Drawing for the job (mm, zero at the part's lowest x, y, z). Round coordinates to 2 decimals unless told otherwise and drop trailing zeros. Write each loop counter-clockwise with the first axis right and the second up, starting at its lowest first coordinate (ties: lowest second). Pieces come first, ordered by that corner, then holes. Notation, with made-up numbers: (53.25, 48) -> (108.25, 48) arc R20 cw to (108.25, 84) -> close; hole circle Ø5 at (77, 39). An arc over 180 degrees is marked (long way). Answer in a Markdown table with one row per item. Add a question column.
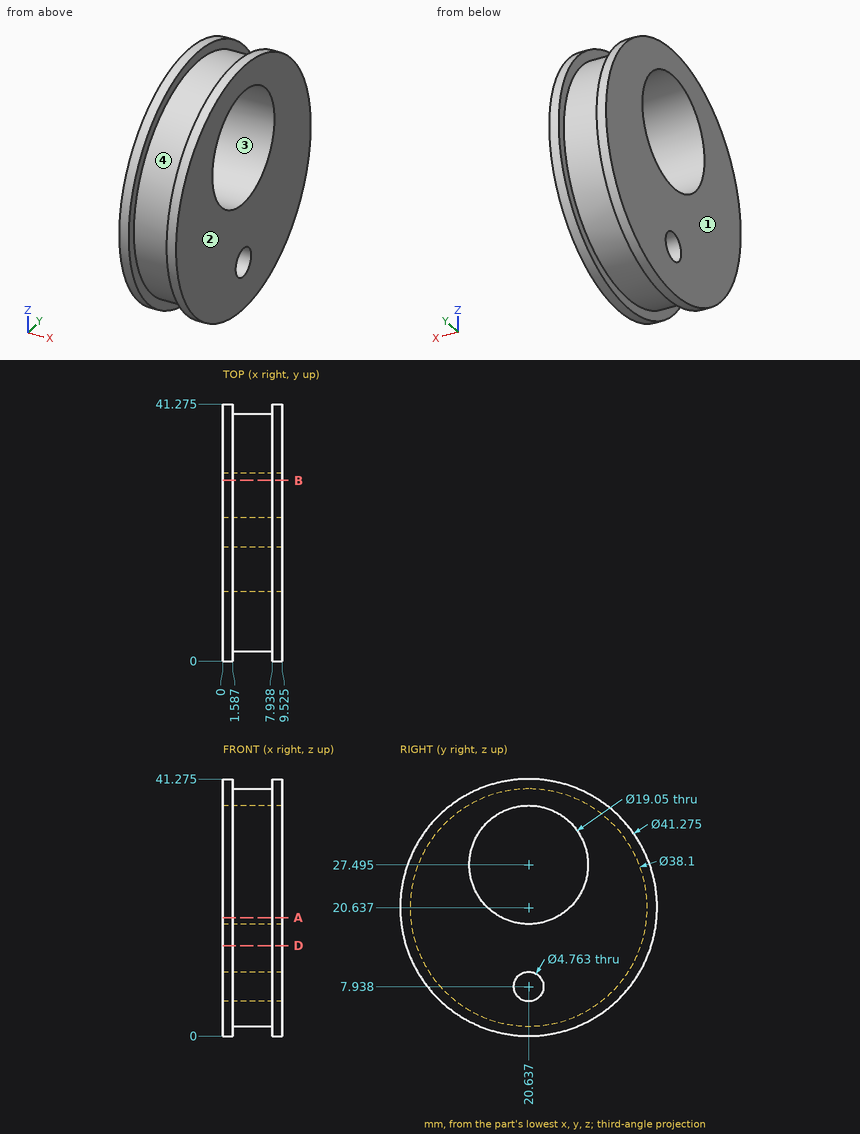
(1) Mould opens along X. For the marked faces 1, 2, 3 and 4 say: pulls with the +X half, pulls with the -X half, needs draft (parallel to the pull), parting line crosses it, or undercut.
(2) Saw through at B-B (y = 29). List the corners of the cut face in (x, z) (1 decimal), plus the area to 3 significant figures.
(3) Probe line 1 along X through (y, z) = (24, 39.5) (1 decimal); line 2 along Z through (x, y) = (2.5, 19) (1 decimal); line 3 along Y through (x, z) = (8, 9.5) (1 decimal). List the from-to ranges inside material, lowest first.
(4) Drop flat-ended pins along their axis: P1, Ø1, axis at x = 6, z = 10.5, coming from the -Y side (1 decimal); P2, Ø4, axis at x = 5.5, z = 4.5, coming from the +Y side (1 decimal); P3, Ø1, axis at x = 5, y = 8, coming from the -Z side (1 decimal). Give the stop position or say it passes through.
(5) Saw through at D-D (z = 14.5). List the corners of the cut face in (x, y) (1 decimal), plus the area to 3 significant figures.
(6) Saw through at A-A (z = 19). List the corners of the cut face in (x, y) (1 decimal).
Answer sheet:
| question | item | result |
|---|---|---|
| 1 | face 1 | pulls with the -X half |
| 1 | face 2 | pulls with the +X half |
| 1 | face 3 | needs draft |
| 1 | face 4 | undercut |
| 2 | outline | (0, 1.8) -> (1.6, 1.8) -> (1.6, 3.5) -> (7.9, 3.5) -> (7.9, 1.8) -> (9.5, 1.8) -> (9.5, 22.9) -> (0, 22.9) -> close; (0, 32.1) -> (9.5, 32.1) -> (9.5, 39.5) -> (7.9, 39.5) -> (7.9, 37.8) -> (1.6, 37.8) -> (1.6, 39.5) -> (0, 39.5) -> close |
| 2 | area | 250 mm² |
| 3 | line 1 | x = 0 to 1.6, 7.9 to 9.5 |
| 3 | line 2 | z = 1.7 to 6.2, 9.7 to 18.1, 36.9 to 39.6 |
| 3 | line 3 | y = 3.3 to 18.8, 22.4 to 38 |
| 4 | P1 | stops at y = 4.2 |
| 4 | P2 | stops at y = 33.4 |
| 4 | P3 | stops at z = 6 |
| 5 | outline | (0, 0.9) -> (1.6, 0.9) -> (1.6, 2.6) -> (7.9, 2.6) -> (7.9, 0.9) -> (9.5, 0.9) -> (9.5, 40.3) -> (7.9, 40.3) -> (7.9, 38.7) -> (1.6, 38.7) -> (1.6, 40.3) -> (0, 40.3) -> close |
| 5 | area | 354 mm² |
| 6 | outline | (0, 0.1) -> (1.6, 0.1) -> (1.6, 1.7) -> (7.9, 1.7) -> (7.9, 0.1) -> (9.5, 0.1) -> (9.5, 16.3) -> (0, 16.3) -> close; (0, 24.9) -> (9.5, 24.9) -> (9.5, 41.2) -> (7.9, 41.2) -> (7.9, 39.6) -> (1.6, 39.6) -> (1.6, 41.2) -> (0, 41.2) -> close |
